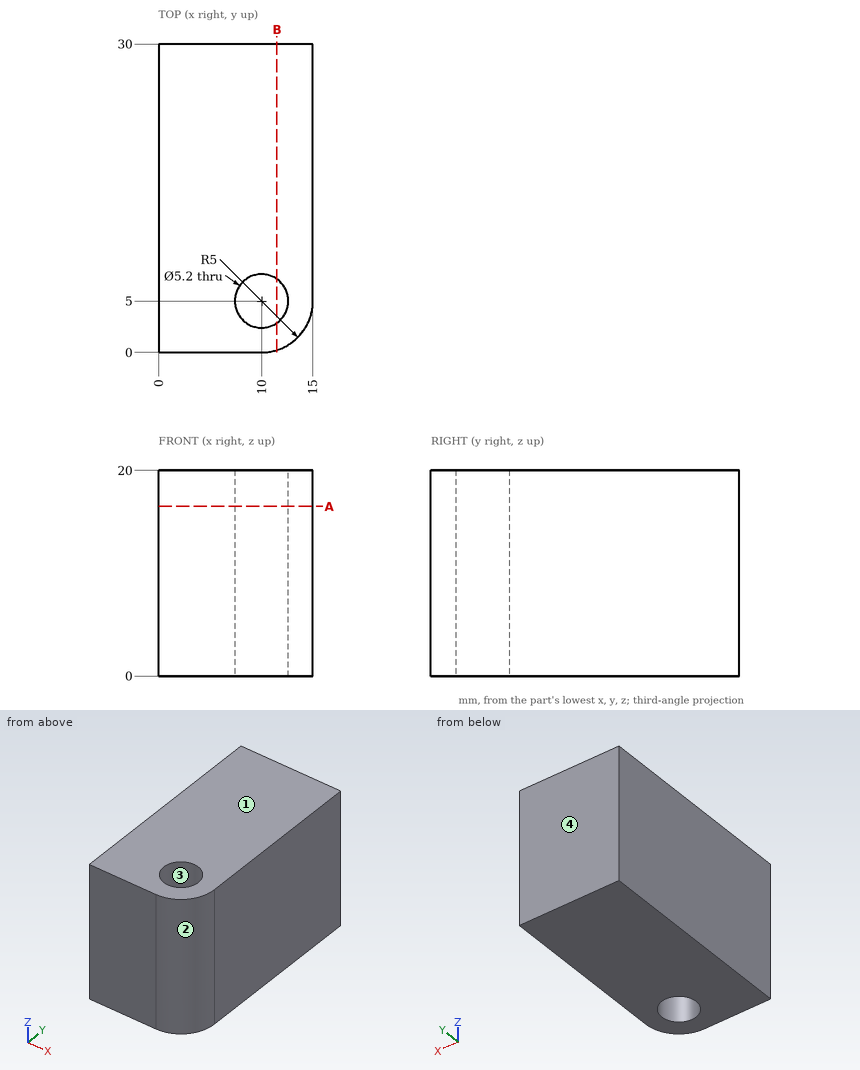
Verification items for this drawing (mm, ordinates from the low corner). Give positions to 0.01 mm unless a question says otherwise; leave off trailing zeros. Write each loop counter-clockwise with the first axis right and the second up, starting at its lowest first coordinate (ties: lowest second). Pieces come first, ordered by that corner, then holes. Notation, with made-up numbers: (32.5, -26) -> (91.5, -26) arc R11 cw to (91.5, -9) -> close; hole circle Ø8 at (38.5, -9). An arc over 180 degrees is marked (long way). Use CSV: the item, a comma, the result in double quotes. Start each with the question number.
Q1. Cross-section at A-A on z = 16.5. Enter the section's corners in (x, y), and give its area (3 significant figures).
Q2. Cross-section at B-B on x = 11.5. Enter the section's corners in (y, z), and give its area (3 significant figures).
Q3. Release check for a two-part mould opening along Y. For the marked faces 1, 2, 3 and 4 record: +Y half, -Y half, draft (parallel to the pull), parting line (faces both ways), or undercut.
Q4. Scan lines: line 1 along Y through (x, z) = (10, 15.5); line 2 along Y through (x, z) = (9.25, 11.5); line 3 along Y through (x, z) = (14.5, 18). Record each from-to range of solid material in increasing order.
Working result:
1,outline,"(0, 0) -> (10, 0) arc R5 ccw to (15, 5) -> (15, 30) -> (0, 30) -> close; hole circle Ø5.2 at (10, 5)"
1,area,"423 mm^2"
2,outline,"(0.23, 0) -> (2.88, 0) -> (2.88, 20) -> (0.23, 20) -> close; (7.12, 0) -> (30, 0) -> (30, 20) -> (7.12, 20) -> close"
2,area,"510 mm^2"
3,face 1,"draft"
3,face 2,"-Y half"
3,face 3,"undercut"
3,face 4,"+Y half"
4,line 1,"y = 0 to 2.4, 7.6 to 30"
4,line 2,"y = 0 to 2.51, 7.49 to 30"
4,line 3,"y = 2.82 to 30"
